Read the model definition and answer for the solid it produces. Units are mm, in the model's axes. Face numbers are marked on the shaded views. Coordinates: 2 decimals unless noted, no trailing zeros. Loops run counter-clockwise (first coordinate to the right, second up) from the corner with the lowest first, then second, coordinate; pieces in that order, holes last. Notation, with made-up numbers: (3.25, 14.5) -> (17.25, 14.5) arc R29 cw to (17.25, 35.5) -> close; hole circle Ø2 at (75, 39). An arc over 180 degrees is marked (long way). Answer in a Markdown table with one row per item.
```python
from build123d import *

# Parameters (mm, degrees)
BOSS_EXTRUDE2_DEPTH = 4
FILLET1_R           = 1
SKETCH3_R           = 1.2
CUT_EXTRUDE1_DEPTH  = 5


with BuildPart() as part:
    # Sketch2 → Boss-Extrude2 (new body)
    with BuildSketch(Plane(origin=(0, 0, 0), x_dir=(1, 0, 0), z_dir=(0, 1, 0))):
        Polygon((3.175426481, 0), (1.58771324, 2.75), (-1.58771324, 2.75), (-3.175426481, 0), (-1.58771324, -2.75), (1.58771324, -2.75), align=None)
    extrude(amount=BOSS_EXTRUDE2_DEPTH)

    # Fillet1
    fillet1_edges = [part.edges().sort_by_distance(p)[0] for p in [
        (0, 4, -2.75),
        (-2.38156986, 4, -1.375),
        (-2.38156986, 4, 1.375),
        (0, 4, 2.75),
        (2.38156986, 4, 1.375),
        (2.38156986, 4, -1.375),
    ]]
    fillet(fillet1_edges, radius=FILLET1_R)

    # Sketch3 → Cut-Extrude1 (cut, through all)
    with BuildSketch(Plane.XZ):
        Circle(SKETCH3_R)
    extrude(amount=-CUT_EXTRUDE1_DEPTH, mode=Mode.SUBTRACT)


solid = part.part
```
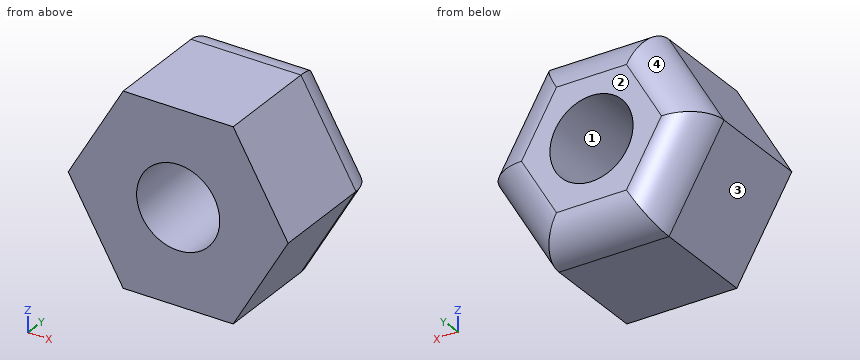
1. A cutting plane is placed at A-A on x = 0. Give the vertices of the cut face in (y, z), and give its area (3 significant figures).
A:
| item | result |
|---|---|
| outline | (0, -2.75) -> (3, -2.75) arc R1 ccw to (4, -1.75) -> (4, -1.2) -> (0, -1.2) -> close; (0, 1.2) -> (4, 1.2) -> (4, 1.75) arc R1 ccw to (3, 2.75) -> (0, 2.75) -> close |
| area | 12.0 mm2 |
2. The mould has two halves that part along Z. Classify the marked faces 1, 2, 3 and 4: pulls with the +Z half, pulls with the -Z half, needs draft (parallel to the pull), parting line crosses it, or undercut.
A:
| item | result |
|---|---|
| face 1 | undercut |
| face 2 | needs draft |
| face 3 | pulls with the -Z half |
| face 4 | pulls with the +Z half |
3. Find the intervals of material crossed by probe 1 along Z at (x, y) = (0, 1.55); probe 2 along X at (y, z) = (1.15, 0.5), in increasing order.
A:
| item | result |
|---|---|
| probe 1 | z = -2.75 to -1.2, 1.2 to 2.75 |
| probe 2 | x = -2.89 to -1.09, 1.09 to 2.89 |
4. A cutting plane is placed at B-B on y = 0.3. Give the vertices of the cut face in (x, z), and give its area (3 significant figures).
A:
| item | result |
|---|---|
| outline | (-3.18, 0) -> (-1.59, -2.75) -> (1.59, -2.75) -> (3.18, 0) -> (1.59, 2.75) -> (-1.59, 2.75) -> close; hole circle Ø2.4 at (0, 0) |
| area | 21.7 mm2 |
